Model file for the job. Use its own axes, mm. A direction names the side the tool comes from. Give positions to 0.01 mm unless a question says otherwise; leave off trailing zeros. Order: outer loops, then holes, each group sorted by start corner. A loop starts at its lowest first (then second) coordinate and runs counter-clockwise, first axis right, second up. Notation, with made-up numbers: (16.5, -34) -> (47.5, -34) arc R25 ccw to (47.5, -5) -> close; hole circle Ø4 at (30.25, 37.25). An arc over 180 degrees is marked (long way). Use CSV: the item, a comma, the result in double quotes. Start each with the question number.
1. Cut at D-D on x = -21. List the corners of the cut face in (y, z).
2. Wall check: line 1 (Y direction, x = -1.25, z = -25); line 2 (Z direction, x = -2.25, y = 8); line 3 (X direction, y = 10.5, z = 21.5). Give the ranges that are in metal, low to high. Write a range as from..to.
3. Pull direction Z, two halves, no side cores. Call faces 3 (the flat face through (-3, 25, -31)), 4 (the flat face through (-2, 13.1, -22.7)), 5 (the flat face through (-5, 25, 28)): released by +Z, released by -Z, zero draft, split by the parting line, or undercut.
4. Cut at A-A on z = -25. List the corners of the cut face in (x, y) (3 decimals).
5. 3-axis set-ups, long thin cutter, end or side, ignore diameter. For faces 1 (the flat face through (-2, 25, 31)), 2 (the flat face through (-6.493, 40.28, 20.976)): which of +Z, -Z, +X, -X, +Y, -Y reach the whole face in a straight line?
6. Cut at B-B on y = 26. List the corners of the cut face in (x, z).
7. Cut at C-C on z = 0. List the corners of the cut face in (x, y), then the cut area to 3 significant figures.
8. Drop flat-ended pins along their axis: pin 1 (4.5 mm diameter, centred on x = -7, z = -25, fed in from +Y); pin 2 (1.5 mm diameter, centred on x = -21.5, y = 11, fed in from +Z); pin 3 (4 mm diameter, centred on y = 13.5, z = 26, fed in from -X); pin 4 (1.5 mm diameter, centred on y = 18, z = -17, fed in from -X). Give the stop position or say it passes through.
```python
from build123d import *

# Parameters (mm, degrees)
BOSS_EXTRUDE1_DEPTH = 50
CUT_EXTRUDE1_DEPTH  = 50
SKETCH2_7_R         = 2.35
CUT_EXTRUDE5_DEPTH  = 10
SKETCH2_10_R        = 2.35
CUT_EXTRUDE8_DEPTH  = 3


with BuildPart() as part:
    # Sketch1 → Boss-Extrude1 (new body)
    with BuildSketch(Plane(origin=(0, 0, 0), x_dir=(1, 0, 0), z_dir=(0, 1, 0))):
        with BuildLine():
            Line((0, -16), (0, -31))
            Line((0, -31), (-5, -31))
            Line((-5, -31), (-5, -23.473389189))
            ThreePointArc((-5, -23.473389189), (-24, 0), (-5, 23.473389189))
            Line((-5, 23.473389189), (-5, 31))
            Line((-5, 31), (0, 31))
            Line((0, 31), (0, 16))
            ThreePointArc((0, 16), (-16, 0), (0, -16))
        make_face()
    extrude(amount=BOSS_EXTRUDE1_DEPTH)

    # Sketch2 → Cut-Extrude1 (cut)
    with BuildSketch(Plane.ZY.offset(5)):
        Polygon((-22.329755005, 33.375), (-19.65951001, 38), (-22.329755005, 42.625), (-27.670244995, 42.625), (-30.34048999, 38), (-27.670244995, 33.375), align=None)
        Polygon((-22.329755005, 7.375), (-19.65951001, 12), (-22.329755005, 16.625), (-27.670244995, 16.625), (-30.34048999, 12), (-27.670244995, 7.375), align=None)
        Polygon((27.670244995, 7.375), (22.329755005, 7.375), (19.65951001, 12), (22.329755005, 16.625), (27.670244995, 16.625), (30.34048999, 12), align=None)
        Polygon((27.670244995, 42.625), (30.34048999, 38), (27.670244995, 33.375), (22.329755005, 33.375), (19.65951001, 38), (22.329755005, 42.625), align=None)
    extrude(amount=CUT_EXTRUDE1_DEPTH, mode=Mode.SUBTRACT)

    # Sketch2_7 → Cut-Extrude5 (cut)
    with BuildSketch(Plane.ZY.offset(5)):
        with BuildLine():
            Line((-23.473389189, 39.786605561), (-23.473389189, 36.213394439))
            ThreePointArc((-23.473389189, 36.213394439), (-22.865751256, 37.016393221), (-22.65, 38))
            ThreePointArc((-22.65, 38), (-22.865751256, 38.983606779), (-23.473389189, 39.786605561))
        make_face()
        with BuildLine():
            ThreePointArc((-23.473389189, 39.786605561), (-27.35, 38), (-23.473389189, 36.213394439))
            Line((-23.473389189, 36.213394439), (-23.473389189, 39.786605561))
        make_face()
        with BuildLine():
            Line((-23.473389189, 10.213394439), (-23.473389189, 13.786605561))
            ThreePointArc((-23.473389189, 13.786605561), (-27.35, 12), (-23.473389189, 10.213394439))
        make_face()
        with BuildLine():
            ThreePointArc((-22.65, 12), (-22.865751256, 12.983606779), (-23.473389189, 13.786605561))
            Line((-23.473389189, 13.786605561), (-23.473389189, 10.213394439))
            ThreePointArc((-23.473389189, 10.213394439), (-22.865751256, 11.016393221), (-22.65, 12))
        make_face()
        with Locations((25, 38)):
            Circle(SKETCH2_7_R)
        with Locations((25, 12)):
            Circle(SKETCH2_7_R)
    extrude(amount=-CUT_EXTRUDE5_DEPTH, mode=Mode.SUBTRACT)

    # Sketch2_10 → Cut-Extrude8 (cut)
    with BuildSketch(Plane.ZY.offset(5)):
        Polygon((-22.329755005, 33.375), (-19.65951001, 38), (-22.329755005, 42.625), (-27.670244995, 42.625), (-30.34048999, 38), (-27.670244995, 33.375), align=None)
        with Locations((-25, 38)):
            Circle(SKETCH2_10_R, mode=Mode.SUBTRACT)
        Polygon((-22.329755005, 7.375), (-19.65951001, 12), (-22.329755005, 16.625), (-27.670244995, 16.625), (-30.34048999, 12), (-27.670244995, 7.375), align=None)
        with Locations((-25, 12)):
            Circle(SKETCH2_10_R, mode=Mode.SUBTRACT)
        Polygon((27.670244995, 7.375), (22.329755005, 7.375), (19.65951001, 12), (22.329755005, 16.625), (27.670244995, 16.625), (30.34048999, 12), align=None)
        with Locations((25, 12)):
            Circle(SKETCH2_10_R, mode=Mode.SUBTRACT)
        Polygon((27.670244995, 42.625), (30.34048999, 38), (27.670244995, 33.375), (22.329755005, 33.375), (19.65951001, 38), (22.329755005, 42.625), align=None)
        with Locations((25, 38)):
            Circle(SKETCH2_10_R, mode=Mode.SUBTRACT)
    extrude(amount=-CUT_EXTRUDE8_DEPTH, mode=Mode.SUBTRACT)


solid = part.part
```
Verdict:
1,outline,"(0, -11.62) -> (50, -11.62) -> (50, 11.62) -> (0, 11.62) -> close"
2,line 1,"0..9.65, 14.35..35.65, 40.35..50"
2,line 2,"-31..-28.03, -21.97..-15.84, 15.84..21.97, 28.03..31"
2,line 3,"-2..0"
3,face 3,"released by -Z"
3,face 4,"undercut"
3,face 5,"zero draft"
4,outline,"(-5, 0) -> (0, 0) -> (0, 9.65) -> (-2, 9.65) -> (-2, 7.375) -> (-5, 7.375) -> close; (-5, 16.625) -> (-2, 16.625) -> (-2, 14.35) -> (0, 14.35) -> (0, 35.65) -> (-2, 35.65) -> (-2, 33.375) -> (-5, 33.375) -> close; (-5, 42.625) -> (-2, 42.625) -> (-2, 40.35) -> (0, 40.35) -> (0, 50) -> (-5, 50) -> close"
5,face 1,"+Z, +X, -X, +Y, -Y"
5,face 2,"-X"
6,outline,"(-5, -31) -> (0, -31) -> (0, -16) arc R16 cw to (0, 16) -> (0, 31) -> (-5, 31) -> (-5, 23.47) arc R24 ccw to (-5, -23.47) -> close"
7,outline,"(-24, 0) -> (-16, 0) -> (-16, 50) -> (-24, 50) -> close"
7,area,"400 mm^2"
8,pin 1,"y = 50"
8,pin 2,"z = 12.06"
8,pin 3,"x = -2"
8,pin 4,"x = -17.66"
